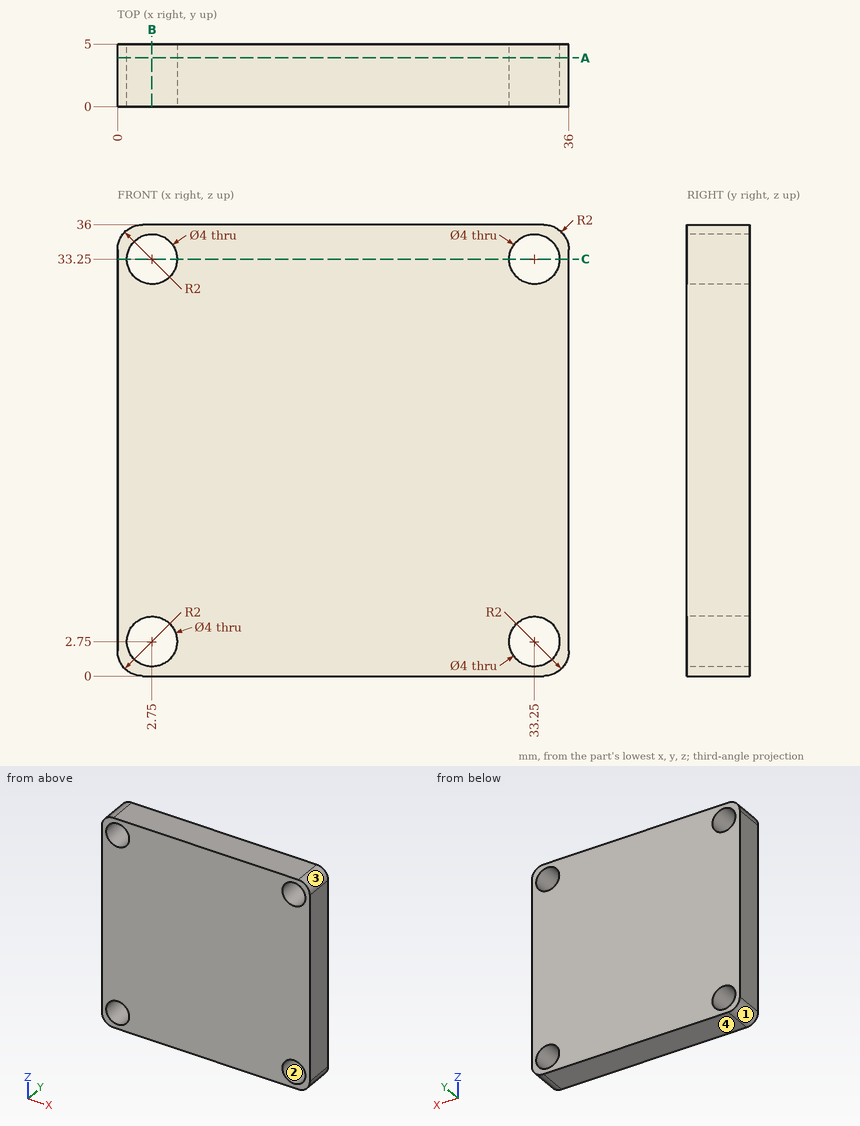
Print and shaded views of the part. All mm, measured from the part's lowest x, y and z. Round coordinates to 2 decimals unless told otherwise and drop trailing zeros. Write each loop counter-clockwise with the first axis right and the second up, starting at its lowest first coordinate (ties: lowest second). Pieces come first, ordered by that corner, then holes. Notation, with made-up numbers: (62, 11.25) -> (111, 11.25) arc R22 ccw to (111, 47.25) -> close; hole circle Ø8 at (71, 29.5). An arc over 180 degrees is marked (long way). Return JSON: item names as keys, results as strings. Group by question number.
Q1. Saw through at C-C on z = 33.25. Write the cut outline in (x, y), plus the area to 3 significant figures.
Q2. Saw through at B-B on x = 2.75. Write the cut outline in (y, z), plus the area to 3 significant figures.
Q3. Mould opens along X. For the marked faces 1, 2, 3 and 4 say: pulls with the +X half, pulls with the -X half, needs draft (parallel to the pull), parting line crosses it, or undercut.
Q4. Saw through at A-A on y = 3.9. Write the cut outline in (x, z).
Q5. Probe L1, parallel to Z at x = 2.75, y = 3.7; L2, parallel to X at y = 1, z = 33; L3, parallel to Z at x = 34.5, y = 4.05. List the from-to ranges inside material, lowest first. Write a range as [from, to].
Answer:
{
 "1": {"outline": "(0, 0) -> (0.75, 0) -> (0.75, 5) -> (0, 5) -> close; (4.75, 0) -> (31.25, 0) -> (31.25, 5) -> (4.75, 5) -> close; (35.25, 0) -> (36, 0) -> (36, 5) -> (35.25, 5) -> close", "area": "140 mm2"},
 "2": {"outline": "(0, 0) -> (5, 0) -> (5, 0.75) -> (0, 0.75) -> close; (0, 4.75) -> (5, 4.75) -> (5, 31.25) -> (0, 31.25) -> close; (0, 35.25) -> (5, 35.25) -> (5, 36) -> (0, 36) -> close", "area": "140 mm2"},
 "3": {"face 1": "pulls with the -X half", "face 2": "undercut", "face 3": "pulls with the +X half", "face 4": "needs draft"},
 "4": {"outline": "(0, 2) arc R2 ccw to (2, 0) -> (34, 0) arc R2 ccw to (36, 2) -> (36, 34) arc R2 ccw to (34, 36) -> (2, 36) arc R2 ccw to (0, 34) -> close; hole circle Ø4 at (2.75, 2.75); hole circle Ø4 at (2.75, 33.25); hole circle Ø4 at (33.25, 2.75); hole circle Ø4 at (33.25, 33.25)"},
 "5": {"L1": "[0, 0.75], [4.75, 31.25], [35.25, 36]", "L2": "[0, 0.77], [4.73, 31.27], [35.23, 36]", "L3": "[0.06, 1.19], [4.31, 31.69], [34.81, 35.94]"}
}
